Autodesk Inventor part; units mm, degrees
ref_plane "Work Plane1" through (29, 0, 0) normal (0, -1, 0) x (1, 0, 0)
ref_plane "YZ Plane" through (0, 0, 0) normal (1, 0, 0) x (0, 1, 0)
ref_plane "XZ Plane" through (0, 0, 0) normal (0, 1, 0) x (-1, 0, 0)
sketch "Sketch1" plane through (0, 0, 0) normal (0, 0, 1) x (1, 0, 0)
  line L0 (-1, 0) -> (30, 0)
  line L1 (30, 0) -> (30, 2)
  line L2 (30, 2) -> (10, 2)
  line L3 (10, 2) -> (9.5705, 2)
  line L4 (9.5705, 2) -> (0, 2)
  line L5 (0, 2) -> (0, 3.5)
  line L6 (0, 3.5) -> (-4, 3.5)
  line L7 (-4, 3.5) -> (-4, 1.7321)
  line L8 (-4, 1.7321) -> (-2, 1.7321)
  line L9 (-2, 1.7321) -> (-1, 0)
  line L10 (-10.8, 0) -> (36.8, 0)
  line L11 (0, -0.7) -> (0, 4.2)
  line L12 (10, 2) -> (0, 2) construction
  dimension "d1" = 20
  dimension "d2" = 0.4295
  dimension "d3" = 4
  dimension "d4" = 2
  dimension "d5" = 60
  dimension "d6" = 4
  dimension "d7" = 4
  dimension "d8" = 3.4641
  dimension "d9" = 7
  dimension "d26" = 30
revolve "Body" add sketch "Sketch1" angle 360 about axis through (-1, 0, 0) along (1, 0, 0)
sketch "Sketch2" plane through (-4, 0, 0) normal (-1, 0, 0) x (0, 0, 1)
  circle A0 centre (0, 0) radius 1.7321
  line L0 (0, -4.9) -> (0, 4.9)
  line L1 (-4.9, 0) -> (4.9, 0)
  line L2 (1.7321, 0) -> (0.866, -1.5)
  line L3 (0.866, -1.5) -> (-0.866, -1.5)
  line L4 (-0.866, -1.5) -> (-1.7321, 0)
  line L5 (-1.7321, 0) -> (-0.866, 1.5)
  line L6 (-0.866, 1.5) -> (0.866, 1.5)
  line L7 (0.866, 1.5) -> (1.7321, 0)
extrude "Slot" add sketch "Sketch2" against normal up to next contours L7 A0 | A0 L2 | L6 L0 A0 | A0 L0 L3 | L0 L6 A0 | A0 L3 L0 | L4 A0 | A0 L5
fillet "Fillet1" radius 0.4 1 edges at (-4, -3.5, 0)
thread "Thread"
chamfer "Chamfer1" distance 0.4294 distance2 0.4294 1 edges at (30, -2, 0) measured on face at (30, -0.499, -0.4421)
ref_plane "Work Plane1" through (29, 0, 0) normal (0, -1, 0) x (1, 0, 0)
fillet "Fillet2" radius 0.1 1 edges at (0, -2, 0)
equation "\"d1\" = GEL"
equation "\"d3\" = KOH"
equation "\"d4\" = INTI"
equation "\"d6\" = GD"
equation "\"d7\" = BDM"
equation "\"d8\" = 1.1547 * SW"
equation "\"d9\" = KOD"
equation "\"d26\" = NLG"
equation "\"d30\" = R"
equation "\"d17\" = RR"
equation "\"d13\" = GEL"
equation "\"d15\" = -0.5 * SPD + 0.5 * GD"
equation "\"d16\" = GUL"
equation "\"GD\" = NND"
equation "\"NLG\" = 30"
equation "\"GEL\" = 20"
equation "\"KOD\" = 7"
equation "\"KOH\" = 4"
equation "\"INTI\" = 2"
equation "\"GAL\" = 0.61345 * PTC"
equation "\"GUL\" = 0.61345 * PTC"
equation "\"BDM\" = NND"
equation "\"SW\" = 3"
equation "\"RR\" = 0.4"
equation "\"SPD\" = 3.14117"
equation "\"R\" = 0.1"
equation "\"TOA\" = 30deg"
equation "\"THREADDIA\" = 4"
equation "\"PTC\" = 0.7"
equation "\"NND\" = 4"
equation "\"E0\" = 1.155 * SW"
equation "\"GD1\" = THREADDIA - 1.2269 * PTC"
properties part number "ANSI B18.3.1M - M4x0.7 x 30" material "Steel, Mild"
Can you work these out from the model? Positions are in its coordinate system, mm. A direction names the side the tool comes from. Give positions to 0.01 mm unless a question says otherwise; leave off trailing zeros. Loops run counter-clockwise (first coordinate to the right, second up) from the corner with the lowest first, then second, coordinate; pieces in that order, holes last. Notation, with made-up numbers: M 75,77 L 83,77 A18 ccw 83,104 Z; hole C 38,79.25 d5. An arc over 180 degrees is marked long. One line per question, with ' | ' between items. Start each with the question number.
Q1. If I drill on line 1 (X direction, y = 0.75, z = 2.75); line 2 (Z direction, x = 10, y = 0.75); line 3 (Y direction, x = 17, z = 1), over which ranges is the centre line in solid material (lowest first)? Write a range as from..to.
Q2. If we mould it in two halves opening along Y, with no side actions, what happens to faces 3 (the flat face through (-2.948, 0.761, 1.293)), 4 (the flat face through (0, 2, -2)), 5 (the cylindrical face through (15, 0, 2))? For each: +Y half, -Y half, draft (parallel to the pull), parting line (faces both ways), or undercut.
Q3. For pin 1 Ø2 at (x, y) = (21, -2) entering from -Z; pin 2 Ø0.5 at (x, z) = (-2.5, -0.5) entering from -Y; pin 3 Ø2 at (x, y) = (13.5, -1) entering from +Z, each with a flat end and sliding along its axis, tell me the tip position at first contact or that it passes through.
Q4. If we section it at A-A (x = 0.5): Please give me the cut outline in (y, z).
Q5. For faces 1 (the cylindrical face through (-1.825, 3.233, 1.341)), 2 (the flat face through (-2.948, 0.74, -1.305)), which set-ups out of +Z, -Z, +X, -X, +Y, -Y let a thin tool reach every point of the face, with its end or its side?
Computed:
1) line 1: x = -4..0 | line 2: z = -1.85..1.85 | line 3: y = -1.73..1.73
2) face 3: undercut | face 4: draft | face 5: parting line
3) pin 1: stops at z = -1.73 | pin 2: stops at y = -3.49 | pin 3: stops at z = 2
4) outline: C 0,0 d4
5) face 1: +X, -X | face 2: -X
